Here's how the part is built. I have some questions about the finished solid (model axes, mm). Face numbers are marked on the shaded views. Round coordinates to 2 decimals unless told otherwise and drop trailing zeros. Write each loop counter-clockwise with the first axis right and the second up, starting at its lowest first coordinate (ties: lowest second). Pieces come first, ordered by that corner, then holes. Notation, with made-up numbers: M 71.5,16.5 L 89.5,16.5 A30 ccw 89.5,44.5 Z; hole C 22.5,16.5 d10. An arc over 180 degrees is marked long. Use a Markdown table: item, result. Add a question column.
Solid Edge part; units mm, degrees
sketch "Sketch1" plane through (0, 0, 0) normal (0, -1, 0) x (1, 0, 0)
  line L0 (-37.6, -25.1) -> (37.6, -25.1)
  line L1 (37.6, -25.1) -> (37.6, 25.1)
  line L2 (37.6, 25.1) -> (-37.6, 25.1)
  line L3 (-37.6, 25.1) -> (-37.6, -25.1)
extrude "Protrusion1" add sketch "Sketch1" along normal mid plane 1
sketch "Sketch2" plane through (0, -0.5, 0) normal (0, -1, 0) x (0, 0, -1)
  circle A0 centre (-22.3, 34.8) radius 1.5
  circle A1 centre (22.3, 34.8) radius 1.5
  circle A2 centre (-22.3, -34.8) radius 1.5
  circle A3 centre (22.3, -34.8) radius 1.5
extrude "Cutout1" cut sketch "Sketch2" against normal up to surface (1 mm away)
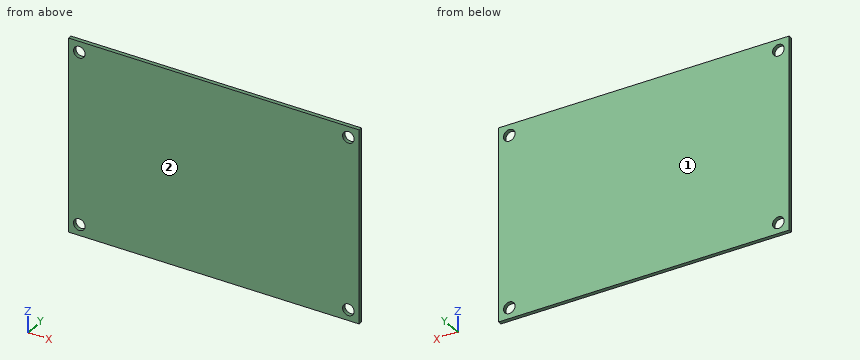
Item 1: For pin 1 Ø2.5 at (x, z) = (34.8, -22.3) entering from -Y; pin 2 Ø3.5 at (x, z) = (-34.8, 22.3) entering from +Y, each with a flat end and sliding along its axis, tell me the tip position at first contact or that it passes through.
Item 2: Imagine slicing it at B-B on x = -34.8. List the corners of the cut face in (y, z) for me, plus the area to 3 significant figures.
Item 3: If we mould it in two halves opening along Y, with no side actions, what happens to the marked faces 1 and 2? For each: +Y half, -Y half, draft (parallel to the pull), parting line (faces both ways), or undercut.
Item 4: I need wall thicknesses on probe 1 along X at (y, z) = (0, 22.3). Which ranges of the line are inside material? Lowest first, please. Write a range as from..to.
Item 5: Imagine slicing it at A-A on z = -22.3. List the corners of the cut face in (x, y) for me.
The answers:
| question | item | result |
|---|---|---|
| 1 | pin 1 | through |
| 1 | pin 2 | y = 0.5 |
| 2 | outline | M -0.5,-25.1 L 0.5,-25.1 L 0.5,-23.8 L -0.5,-23.8 Z; M -0.5,-20.8 L 0.5,-20.8 L 0.5,20.8 L -0.5,20.8 Z; M -0.5,23.8 L 0.5,23.8 L 0.5,25.1 L -0.5,25.1 Z |
| 2 | area | 44.2 mm² |
| 3 | face 1 | +Y half |
| 3 | face 2 | -Y half |
| 4 | probe 1 | -37.6..-36.3, -33.3..33.3, 36.3..37.6 |
| 5 | outline | M -37.6,-0.5 L -36.3,-0.5 L -36.3,0.5 L -37.6,0.5 Z; M -33.3,-0.5 L 33.3,-0.5 L 33.3,0.5 L -33.3,0.5 Z; M 36.3,-0.5 L 37.6,-0.5 L 37.6,0.5 L 36.3,0.5 Z |
